Verification items for the finished model (mm, model axes). A direction names the side the tool comes from. Coordinates: 2 decimals unless noted, no trailing zeros. Order: outer loops, then holes, each group sorted by start corner. A loop starts at its lowest first (then second) coordinate and runs counter-clockwise, first axis right, second up. Notation, with made-up numbers: (81, 20.5) -> (91, 20.5) arc R19 cw to (91, 42.5) -> close; hole circle Ø1 at (38.25, 52). An arc over 180 degrees is marked (long way). Write each question's results on one line, items separated by ' | '. Start each with the question number.
(1) Set-up check for faces 4 (the flat face through (4.513, -1.476, -7.246)), 5 (the flat face through (-7, 0, -5.5)), 6 (the flat face through (0.8, -9, -6.5)): record each of +Z, -Z, +X, -X, +Y, -Y from which the full face is reachable in a straight line by a thin tool's end or side.
(2) Cross-section at A-A on x = -10.5. Enter the section's corners in (y, z).
(3) Cross-section at C-C on x = -15.5. Enter the section's corners in (y, z), and give its area (3 significant figures).
(4) Draft check along Y on faces 1 (the flat face through (0, 8.5, -2)), 2 (the flat face through (-21.44, -0.119, -6.993)), 3 (the flat face through (-16, 15.5, -2)). Enter one of: +Y half, -Y half, draft (parallel to the pull), parting line (faces both ways), or undercut.
(5) Go/stop test with flat-tipped pins: pin 1 (3.5 mm diameter, centred on y = -13.5, z = -1, fed in from -X); pin 2 (0.5 mm diameter, centred on x = 16, z = -0.5, fed in from +Y); pin 3 (1.2 mm diameter, centred on x = -21, y = 0.5, fed in from +Z). Record where each tip stops, or that it passes through.
(6) Cross-section at B-B on y = 12. Enter the section's corners in (x, z), and give its area (3 significant figures).
(7) Thickness scan on probe 1 along Y at (x, z) = (-17, -0.5); probe 2 along Y at (x, z) = (11, -0.75); probe 3 along X at (y, z) = (0, -4.7) (1 decimal). Record the ranges inside material, lowest first. Write a range as [from, to].
```python
from build123d import *

# Parameters (mm, degrees)
PAD004_DEPTH            = 8.5
SKETCH014_W             = 34.267
SKETCH014_H             = 17
POCKET008_DEPTH         = 5.5
SKETCH015_W             = 6
SKETCH015_H             = 20
POCKET009_DEPTH         = 5.5
SKETCH016_W             = 4.3
SKETCH016_H             = 3.5
POCKET010_DEPTH         = 3
SKETCH017_R             = 1.25
POCKET011_DEPTH         = 35.768
CHAMFER007_SIZE         = 1.49999
POCKET012_DEPTH         = 5.5
CHAMFER008_SIZE         = 4
SKETCH019_W             = 17
SKETCH019_H             = 2
PAD005_DEPTH            = 1.2
SKETCH020_W             = 17
SKETCH020_H             = 3
PAD006_DEPTH            = 1.5
CHAMFER009_SIZE         = 2
SKETCH021_R             = 3
PAD007_DEPTH            = 4.6
FILLET001_R             = 3
CHAMFER010_SIZE         = 3
CHAMFER011_SIZE         = 1
CHAMFER012_SIZE         = 2
SKETCH022_W             = 71.294541
SKETCH022_H             = 63.230997
POCKET013_DEPTH         = 1
SKETCH023_R             = 1.6
POCKET014_DEPTH         = 6.601
POCKET015_DEPTH         = 3
CHAMFER013_SIZE         = 0.5
CHAMFER015_SIZE         = 1
FILLET002_R             = 1
SKETCH028_R             = 1.6
POCKET018_DEPTH         = 2
SKETCH029_W             = 12
SKETCH029_H             = 1
POCKET019_DEPTH         = 5
POCKET019_FACE86_R      = 1.6
PAD010_DEPTH            = 1
PAD010_FACE85_R         = 1.6
POCKET022_DEPTH         = 0.3
BODY001_PLACEMENT_ANGLE = 180


with BuildPart() as part:
    # Sketch013 → Pad004 (new body)
    with BuildSketch(Plane.XY):
        Polygon((-11.7335, -10), (16.5335, -10), (16.5335, 10), (-11.7335, 10), (-11.7335, 15.5), (-19.2335, 15.5), (-19.2335, -15.5), (-11.7335, -15.5), align=None)
    extrude(amount=PAD004_DEPTH)

    # Sketch014 (on Face9 of Pad004) → Pocket008 (cut)
    with BuildSketch(Plane(origin=(0, 0, 0), x_dir=(1, 0, 0), z_dir=(0, 0, -1))):
        with Locations((-2.1, 0)):
            Rectangle(SKETCH014_W, SKETCH014_H)
    extrude(amount=-POCKET008_DEPTH, mode=Mode.SUBTRACT)

    # Sketch015 (on Face4 of Pocket008) → Pocket009 (cut)
    with BuildSketch(Plane(origin=(0, 0, 0), x_dir=(1, 0, 0), z_dir=(0, 0, -1))):
        with Locations((-16.2335, 0)):
            Rectangle(SKETCH015_W, SKETCH015_H)
    extrude(amount=-POCKET009_DEPTH, mode=Mode.SUBTRACT)

    # Sketch016 (on Face4 of Pocket009) → Pocket010 (cut)
    with BuildSketch(Plane(origin=(0, 0, 0), x_dir=(1, 0, 0), z_dir=(0, 0, -1))):
        with Locations((-16.0835, 12.75)):
            Rectangle(SKETCH016_W, SKETCH016_H)
    pocket010 = extrude(amount=-POCKET010_DEPTH, mode=Mode.SUBTRACT)

    # Mirrored002: Pocket010 across Sketch016 H_Axis
    add(pocket010.mirror(Plane(origin=(0, 0, 0), x_dir=(0, 0, -1), z_dir=(0, -1, 0))), mode=Mode.SUBTRACT)

    # Sketch017 (on Face8 of Mirrored002) → Pocket011 (cut, through all)
    with BuildSketch(Plane(origin=(-19.2335, 0, 0), x_dir=(0, -1, 0), z_dir=(-1, 0, 0))):
        with Locations((12.495, 0)):
            Circle(SKETCH017_R)
        with Locations((-12.495, 0)):
            Circle(SKETCH017_R)
    extrude(amount=-POCKET011_DEPTH, mode=Mode.SUBTRACT)

    # Chamfer007
    chamfer007_edges = [part.edges().sort_by_distance(p)[0] for p in [
        (-13.2335, 10, 2.75),
        (-13.2335, -10, 2.75),
    ]]
    chamfer(chamfer007_edges, length=CHAMFER007_SIZE)

    # Sketch018 (on Face8 of Pocket011) → Pocket012 (cut)
    with BuildSketch(Plane.XZ.offset(15.5)):
        Polygon((-11.7335, 3.6), (-13.4335, 5.3), (-13.4335, 8.5), (-11.7335, 8.5), align=None)
    pocket012 = extrude(amount=-POCKET012_DEPTH, mode=Mode.SUBTRACT)

    # Mirrored003: Pocket012 across XZ
    add(pocket012.mirror(Plane.XZ), mode=Mode.SUBTRACT)

    # Chamfer008
    chamfer008_edges = [part.edges().sort_by_distance(p)[0] for p in [
        (-16.3335, -15.5, 8.5),
        (-16.3335, 15.5, 8.5),
    ]]
    chamfer(chamfer008_edges, length=CHAMFER008_SIZE)

    # Sketch019 (on Face1 of Chamfer008) → Pad005 (join)
    with BuildSketch(Plane(origin=(-19.2335, 0, 0), x_dir=(0, -1, 0), z_dir=(-1, 0, 0))):
        with Locations((0, 7.5)):
            Rectangle(SKETCH019_W, SKETCH019_H)
    extrude(amount=PAD005_DEPTH)

    # Sketch020 (on Face23 of Pad005) → Pad006 (join)
    with BuildSketch(Plane(origin=(-20.4335, 0, 0), x_dir=(0, -1, 0), z_dir=(-1, 0, 0))):
        with Locations((0, 7)):
            Rectangle(SKETCH020_W, SKETCH020_H)
    extrude(amount=PAD006_DEPTH)

    # Chamfer009
    chamfer009_edges = [part.edges().sort_by_distance(p)[0] for p in [
        (-21.9335, 0, 8.5),
    ]]
    chamfer(chamfer009_edges, length=CHAMFER009_SIZE)

    # Sketch021 → Pad007 (join)
    with BuildSketch(Plane(origin=(0, 0, 5.5), x_dir=(1, 0, 0), z_dir=(0, 0, -1))):
        with Locations((1.905, 0)):
            Circle(SKETCH021_R)
    extrude(amount=PAD007_DEPTH)

    # Fillet001
    fillet001_edges = [part.edges().sort_by_distance(p)[0] for p in [
        (-1.095, 0, 5.5),
    ]]
    fillet(fillet001_edges, radius=FILLET001_R)

    # Chamfer010
    chamfer010_edges = [part.edges().sort_by_distance(p)[0] for p in [
        (1.55, -10, 8.5),
        (16.5335, 0, 8.5),
        (1.55, 10, 8.5),
    ]]
    chamfer(chamfer010_edges, length=CHAMFER010_SIZE)

    # Chamfer011
    chamfer011_edges = [part.edges().sort_by_distance(p)[0] for p in [
        (15.0335, -8.5, 2.75),
        (15.0335, 8.5, 2.75),
    ]]
    chamfer(chamfer011_edges, length=CHAMFER011_SIZE)

    # Chamfer012
    chamfer012_edges = [part.edges().sort_by_distance(p)[0] for p in [
        (16.5335, -10, 2.75),
        (16.5335, 10, 2.75),
    ]]
    chamfer(chamfer012_edges, length=CHAMFER012_SIZE)

    # Sketch022 (on Face47 of Chamfer012) → Pocket013 (cut)
    with BuildSketch(Plane.XY.offset(8.5)):
        with Locations((3.279843, 6.184065)):
            Rectangle(SKETCH022_W, SKETCH022_H)
    extrude(amount=-POCKET013_DEPTH, mode=Mode.SUBTRACT)

    # Sketch023 (on Face59 of Pocket013) → Pocket014 (cut, through all)
    with BuildSketch(Plane(origin=(0, 0, 0.9), x_dir=(1, 0, 0), z_dir=(0, 0, -1))):
        with Locations((1.905, 0)):
            Circle(SKETCH023_R)
    extrude(amount=-POCKET014_DEPTH, mode=Mode.SUBTRACT)

    # Sketch024 (on Face47 of Pocket014) → Pocket015 (cut)
    with BuildSketch(Plane.XY.offset(7.5)):
        Polygon((3.492713, 2.75), (0.317287, 2.75), (-1.270426, 0), (0.317287, -2.75), (3.492713, -2.75), (5.080426, 0), align=None)
    extrude(amount=-POCKET015_DEPTH, mode=Mode.SUBTRACT)

    # Chamfer013
    chamfer013_edges = [part.edges().sort_by_distance(p)[0] for p in [
        (4.28657, 1.375, 7.5),
        (1.905, 2.75, 7.5),
        (-0.47657, 1.375, 7.5),
        (-0.47657, -1.375, 7.5),
        (1.905, -2.75, 7.5),
        (4.28657, -1.375, 7.5),
    ]]
    chamfer(chamfer013_edges, length=CHAMFER013_SIZE)

    # Chamfer015
    chamfer015_edges = [part.edges().sort_by_distance(p)[0] for p in [
        (0.4, 8.5, 5.5),
        (14.5335, 8, 5.5),
        (15.0335, 0, 5.5),
        (0.4, -8.5, 5.5),
        (14.5335, -8, 5.5),
    ]]
    chamfer(chamfer015_edges, length=CHAMFER015_SIZE)

    # Fillet002
    fillet002_edges = [part.edges().sort_by_distance(p)[0] for p in [
        (-16.983495, 10, 5.5),
        (-16.983495, -10, 5.5),
    ]]
    fillet(fillet002_edges, radius=FILLET002_R)

    # Sketch028 (on Face5 of Fillet002) → Pocket018 (cut)
    with BuildSketch(Plane(origin=(-19.2335, 0, 0), x_dir=(0, -1, 0), z_dir=(-1, 0, 0))):
        with Locations((-12.495, 0)):
            Circle(SKETCH028_R)
        with Locations((12.495, 0)):
            Circle(SKETCH028_R)
    extrude(amount=-POCKET018_DEPTH, mode=Mode.SUBTRACT)

    # Sketch029 (on Face49 of Pocket018) → Pocket019 (cut)
    with BuildSketch(Plane.YZ.offset(16.5335)):
        with Locations((0, 0.5)):
            Rectangle(SKETCH029_W, SKETCH029_H)
    extrude(amount=-POCKET019_DEPTH, mode=Mode.SUBTRACT)

    # Pocket019 Face86 → Pad010 (add)
    with BuildSketch(Plane(origin=(1.905, 0, 4.5), x_dir=(0, 1, 0), z_dir=(0, 0, 1))):
        Polygon((2.75, -1.587713), (2.75, 1.587713), (0, 3.175426), (-2.75, 1.587713), (-2.75, -1.587713), (0, -3.175426), align=None)
        Circle(POCKET019_FACE86_R, mode=Mode.SUBTRACT)
    extrude(amount=PAD010_DEPTH)

    # Pad010 Face85 → Pocket022 (cut)
    with BuildSketch(Plane(origin=(1.905, 0, 5.5), x_dir=(0, 1, 0), z_dir=(0, 0, 1))):
        Polygon((2.75, -1.587713), (2.75, 1.587713), (0, 3.175426), (-2.75, 1.587713), (-2.75, -1.587713), (0, -3.175426), align=None)
        Circle(PAD010_FACE85_R, mode=Mode.SUBTRACT)
    extrude(amount=-POCKET022_DEPTH, mode=Mode.SUBTRACT)


with BuildPart() as part_1:
    # Body001 placement: moved
    add(part.part.rotate(Axis((0, 0, 0), (1, 0, 0)), BODY001_PLACEMENT_ANGLE))


solid = part_1.part
```
Results are:
1) face 4: -Z | face 5: +Z | face 6: -Z, +X, -Y
2) outline: (-10, -5.5) -> (-8, -7.5) -> (8, -7.5) -> (10, -5.5) -> (10, 0) -> (8.5, 0) -> (8.5, -4.5) -> (7.5, -5.5) -> (-7.5, -5.5) -> (-8.5, -4.5) -> (-8.5, 0) -> (-10, 0) -> close
3) outline: (-15.5, -4.5) -> (-12.5, -7.5) -> (12.5, -7.5) -> (15.5, -4.5) -> (15.5, 0) -> (14.5, 0) -> (14.5, -3) -> (11, -3) -> (11, 0) -> (10, 0) -> (10, -4.5) arc R1 cw to (9, -5.5) -> (-9, -5.5) arc R1 cw to (-10, -4.5) -> (-10, 0) -> (-11, 0) -> (-11, -3) -> (-14.5, -3) -> (-14.5, 0) -> (-15.5, 0) -> close | area: 92.9 mm2
4) face 1: undercut | face 2: draft | face 3: +Y half
5) pin 1: stops at x = -19.23 | pin 2: stops at y = 8.78 | pin 3: stops at z = -5.5
6) outline: (-19.23, -7.5) -> (-13.43, -7.5) -> (-13.43, -5.3) -> (-11.73, -3.6) -> (-11.73, -1.15) -> (-13.93, -1.15) -> (-13.93, -3) -> (-18.23, -3) -> (-18.23, -1.52) -> (-19.23, -1.52) -> close | area: 34.1 mm2
7) probe 1: y = [-15.5, -14.5], [-11, -10], [10, 11], [14.5, 15.5] | probe 2: y = [-10, -8.5], [8.5, 10] | probe 3: x = [-2.1, 0.3], [3.5, 5.9], [14.8, 16.5]
